For this review, take the finished solid that the model builds, in its own axes (mm). A direction names the side the tool comes from. Give positions to 0.01 mm unless a question says otherwise; leave off trailing zeros.
from build123d import *

# Parameters (mm, degrees)
F2_R = 2
F3_R = 2


with BuildPart() as f1:
    # F0 (on Front) → F1 (revolve)
    with BuildSketch(Plane.XZ):
        Polygon((0, 18.25), (0, 4), (5.25, 4), (5.25, 23.25), (4, 23.25), (2.5, 18.25), align=None)
        Polygon((-5.25, 4), (0, 4), (0, 18.25), (-2.5, 18.25), (-4, 23.25), (-5.25, 23.25), align=None)
    revolve(axis=Axis((0.717638, 0, 0), (1, 0, 0)))

    # F2
    f2_edges = [f1.edges().sort_by_distance(p)[0] for p in [
        (2.5, 0, -18.25),
    ]]
    fillet(f2_edges, radius=F2_R)

    # F3
    f3_edges = [f1.edges().sort_by_distance(p)[0] for p in [
        (-2.5, 0, -18.25),
    ]]
    fillet(f3_edges, radius=F3_R)


solid = f1.part
(1) Clearance check with flat-ended pins moving along their axes: pin 1 Ø3 at (x, z) = (-3, 0.5) entering from +Y; pin 2 Ø2 at (x, y) = (0.5, -3) entering from +Z. State where each tip first meets the part, or that it passes through.
(2) Tool access review of faces 4 (the conical face through (2.98, 12.08, -15.75)), 5 (the flat face through (5.25, 5, 0)): name each direction out of +Z, -Z, +X, -X, +Y, -Y from which nothing blocks a thin tool from reaching the whole face with its end or side.
(3) The part is to be moulded in two halves that separate along Y. For faces 1 (the flat face through (-5.25, 5, 0)), 2 (the cylindrical face through (-4.634, -6.984, 22.176)), 3 (the cylindrical face through (0.074, 3.905, -0.867)), say which applies: +Y half, -Y half, draft (parallel to the pull), parting line (faces both ways), or undercut.
(4) For L1, parallel to Y at x = 0.75, z = 0; L2, parallel to Z at x = -1.75, y = 0, list the stretches that pass through material, from the lowest coordinate up.
The answers:
1. pin 1: stops at y = 23.25
1. pin 2: stops at z = 18.14
2. face 4: none
2. face 5: +Z, -Z, +X, +Y, -Y
3. face 1: draft
3. face 2: parting line
3. face 3: undercut
4. L1: y = -18.25 to -4, 4 to 18.25
4. L2: z = -18.39 to -4, 4 to 18.39
